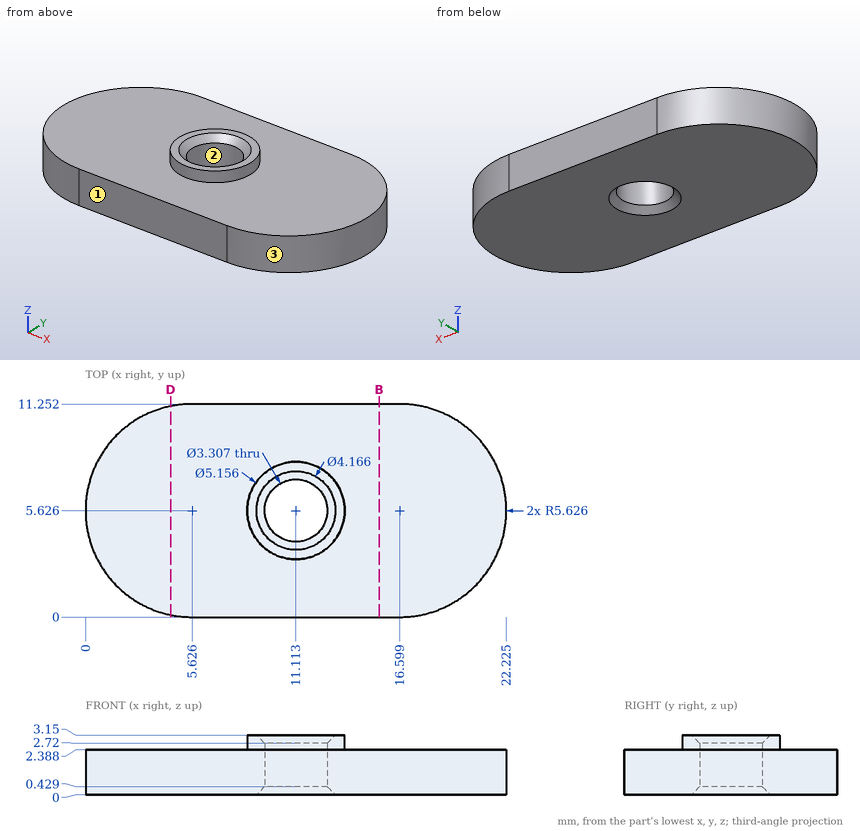
The drawing under review shows one solid part. Ordinate dimensions are in mm from its lowest x, y, z. Round coordinates to 2 decimals unless told otherwise and drop trailing zeros. Write each loop counter-clockwise with the first axis right and the second up, starting at its lowest first coordinate (ties: lowest second). Pieces come first, ordered by that corner, then holes. Notation, with made-up numbers: (14.25, 68) - (41.25, 68) arc R18 cw to (41.25, 91) - close; hole circle Ø9 at (36, 54). An arc over 180 degrees is marked (long way). Put each result on its own line as item: value.
Q1. We need section D-D (x = 4.5). Give the boundary of the cut face in (y, z), and give its area (3 significant figures).
Solved:
outline: (0.11, 0) - (11.14, 0) - (11.14, 2.39) - (0.11, 2.39) - close
area: 26.3 mm2
Q2. Mouldability with a two-part tool opening along X and no side actions: class the marked faces 1, 2 and 3 as released by +X, released by -X, zero draft, split by the parting line, or undercut.
Solved:
face 1: zero draft
face 2: undercut
face 3: released by +X
Q3. Wall thickness on probe 1 along Z at (x, y) = (4, 1.25); probe 2 along X at (y, z) = (6, 1.1); probe 3 along X at (y, z) = (6.5, 2.9) (1 decimal): over which ranges is each line inside the solid? List them lowest first.
Solved:
probe 1: z = 0 to 2.39
probe 2: x = 0.01 to 9.5, 12.72 to 22.21
probe 3: x = 8.7 to 9.5, 12.7 to 13.5
Q4. We need section B-B (x = 15.5). Give the boundary of the cut face in (y, z).
Solved:
outline: (0, 0) - (11.25, 0) - (11.25, 2.39) - (0, 2.39) - close
